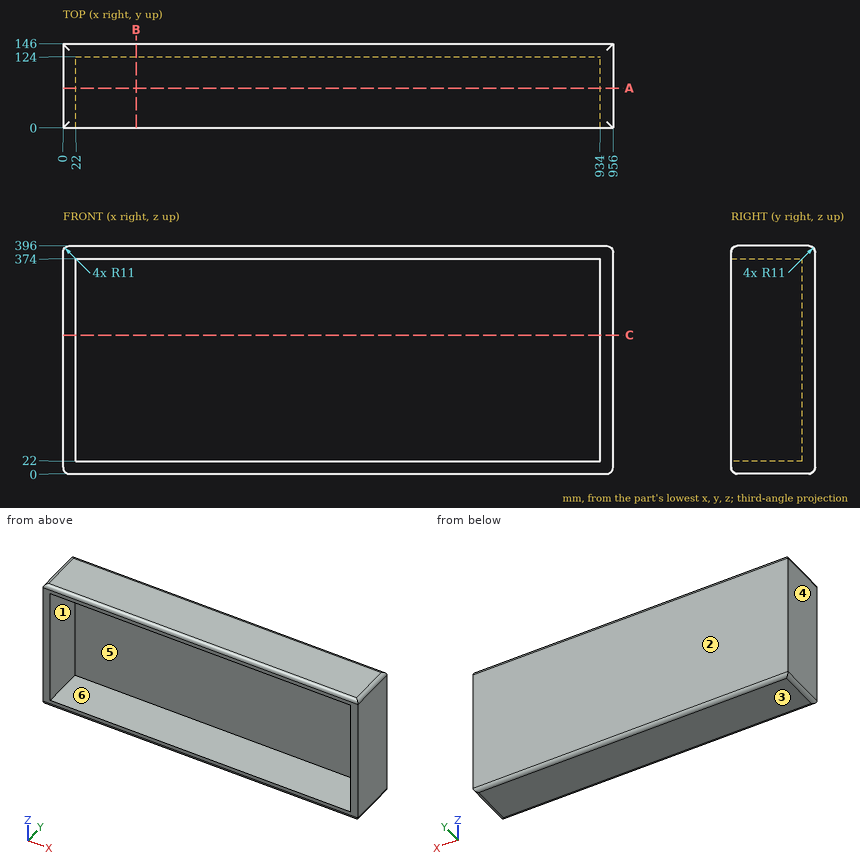
Geometry check sheet. Reference: drawing and pictorial views, mm from the part's lowest x, y, z. A direction names the side the tool comes from. Give positions to 0.01 mm unless a question says otherwise; leave off trailing zeros. Order: outer loops, then holes, each group sorted by start corner. A loop starts at its lowest first (then second) coordinate and runs counter-clockwise, first axis right, second up. Notation, with made-up numbers: M -30,-27 L 5,-27 A26 ccw 5,1 Z; hole C -33.75,38 d2. An arc over 180 degrees is marked long. Answer as CSV lines item,"result". Start each with the question number.
Item 1: Cross-section at A-A on y = 69.5. Enter the section's corners in (x, z).
Item 2: Cross-section at B-B on x = 127. Enter the section's corners in (y, z), plus the area to 3 significant figures.
Item 3: Cross-section at C-C on z = 241. Enter the section's corners in (x, y), plus the area to 3 significant figures.
Item 4: Thickness scan on line 1 (X direction, y = 67.5, z = 324); line 2 (Z direction, x = 124, y = 33.5); line 3 (Z direction, x = 810.5, y = 9.5). Record the ranges inside material, lowest first. Write a range as [from, to].
Item 5: Tool access check on the marked faces 1 and 2. Record the directions out of +Z, -Z, +X, -X, +Y, -Y that give a thin tool (end or side, any length) a straight path to the whole face; none if there is none.
Item 6: Mould release check, pull along Z, two halves, no side actions. Record for the marked faces 3, 4, 5 and 6: +Z half, -Z half, draft (parallel to the pull), parting line (faces both ways), or undercut.
Item 7: Gauge pin test, flat end, axial feed: P1, Ø12, axis at x = 739.5, z = 278, coming from the -Y side. Record the tip position at first contact, or that the pin passes through.
Established:
1,outline,"M 0,11 A11 ccw 11,0 L 945,0 A11 ccw 956,11 L 956,385 A11 ccw 945,396 L 11,396 A11 ccw 0,385 Z; hole M 22,22 L 934,22 L 934,374 L 22,374 Z"
2,outline,"M 0,11 A11 ccw 11,0 L 135,0 A11 ccw 146,11 L 146,385 A11 ccw 135,396 L 11,396 A11 ccw 0,385 L 0,374 L 124,374 L 124,22 L 0,22 Z"
2,area,"14,100 mm^2"
3,outline,"M 0,0 L 22,0 L 22,124 L 934,124 L 934,0 L 956,0 L 956,146 L 0,146 Z"
3,area,"26,500 mm^2"
4,line 1,"x = [0, 22], [934, 956]"
4,line 2,"z = [0, 22], [374, 396]"
4,line 3,"z = [0.1, 22], [374, 395.9]"
5,face 1,"-Y"
5,face 2,"+Z, -Z, +X, -X, +Y"
6,face 3,"-Z half"
6,face 4,"draft"
6,face 5,"undercut"
6,face 6,"undercut"
7,P1,"stops at y = 124"
